The listing builds one solid part. Answer for the finished solid, in the listing's coordinates (mm). A direction names the side the tool comes from. Round coordinates to 2 decimals unless told otherwise and drop trailing zeros. Loops run counter-clockwise (first coordinate to the right, second up) from the corner with the lowest first, then second, coordinate; pieces in that order, holes last. Notation, with made-up numbers: (3, 86.25) - (19, 86.25) arc R19 ccw to (19, 102.25) - close; hole circle Ø1 at (7, -36.75). An arc over 180 degrees is marked (long way). One line per item, written item: value.
```python
from build123d import *

# Parameters (mm, degrees)
SKETCH1_W           = 155
SKETCH1_H           = 155
SKETCH1_R           = 1.5
SKETCH1_W_2         = 85
SKETCH1_H_2         = 85
BOSS_EXTRUDE1_DEPTH = 8
SKETCH3_W           = 128
SKETCH3_H           = 128
CUT_EXTRUDE2_DEPTH  = 2.85
FILLET1_R           = 3
SKETCH4_R           = 2.5
CUT_EXTRUDE3_DEPTH  = 2.5
SKETCH5_R           = 1.75
CUT_EXTRUDE4_DEPTH  = 23
SKETCH6_R           = 3.35
CUT_EXTRUDE5_DEPTH  = 3.5


with BuildPart() as part:
    # Sketch1 → Boss-Extrude1 (new body)
    with BuildSketch(Plane.XY):
        Rectangle(SKETCH1_W, SKETCH1_H)
        with Locations((-50, 50)):
            Circle(SKETCH1_R, mode=Mode.SUBTRACT)
        with Locations((50, 50)):
            Circle(SKETCH1_R, mode=Mode.SUBTRACT)
        with Locations((50, -50)):
            Circle(SKETCH1_R, mode=Mode.SUBTRACT)
        with Locations((-50, -50)):
            Circle(SKETCH1_R, mode=Mode.SUBTRACT)
        Rectangle(SKETCH1_W_2, SKETCH1_H_2, mode=Mode.SUBTRACT)
    extrude(amount=BOSS_EXTRUDE1_DEPTH)

    # Sketch3 → Cut-Extrude2 (cut)
    with BuildSketch(Plane.XY.offset(8)):
        Rectangle(SKETCH3_W, SKETCH3_H)
    extrude(amount=-CUT_EXTRUDE2_DEPTH, mode=Mode.SUBTRACT)

    # Fillet1
    fillet1_edges = [part.edges().sort_by_distance(p)[0] for p in [
        (77.5, -77.5, 4),
        (-77.5, -77.5, 4),
        (-77.5, 77.5, 4),
        (77.5, 77.5, 4),
    ]]
    fillet(fillet1_edges, radius=FILLET1_R)

    # Sketch4 → Cut-Extrude3 (cut)
    with BuildSketch(Plane(origin=(0, 0, 5.15), x_dir=(-1, 0, 0), z_dir=(0, 0, -1))):
        with Locations((-50, 50)):
            Circle(SKETCH4_R)
        with Locations((50, 50)):
            Circle(SKETCH4_R)
        with Locations((50, -50)):
            Circle(SKETCH4_R)
        with Locations((-50, -50)):
            Circle(SKETCH4_R)
    extrude(amount=CUT_EXTRUDE3_DEPTH, mode=Mode.SUBTRACT)

    # Sketch5 → Cut-Extrude4 (cut)
    with BuildSketch(Plane.XY.offset(8)):
        with Locations((0, 69.431322576)):
            Circle(SKETCH5_R)
        with Locations((-69.610191061, 69.610191061)):
            Circle(SKETCH5_R)
        with Locations((69.431322576, 0)):
            Circle(SKETCH5_R)
        with Locations((69.610191061, 69.610191061)):
            Circle(SKETCH5_R)
        with Locations((0, -69.431322576)):
            Circle(SKETCH5_R)
        with Locations((69.610191061, -69.610191061)):
            Circle(SKETCH5_R)
        with Locations((-69.431322576, 0)):
            Circle(SKETCH5_R)
        with Locations((-69.610191061, -69.610191061)):
            Circle(SKETCH5_R)
    extrude(amount=-CUT_EXTRUDE4_DEPTH, mode=Mode.SUBTRACT)

    # Sketch6 → Cut-Extrude5 (cut)
    with BuildSketch(Plane(origin=(0, 0, 0), x_dir=(-1, 0, 0), z_dir=(0, 0, -1))):
        with Locations((-69.610191061, 69.610191061)):
            Circle(SKETCH6_R)
        with Locations((69.610191061, 69.610191061)):
            Circle(SKETCH6_R)
        with Locations((69.610191061, -69.610191061)):
            Circle(SKETCH6_R)
        with Locations((-69.610191061, -69.610191061)):
            Circle(SKETCH6_R)
        with Locations((-69.431322576, 0)):
            Circle(SKETCH6_R)
        with Locations((0, 69.431322576)):
            Circle(SKETCH6_R)
        with Locations((69.431322576, 0)):
            Circle(SKETCH6_R)
        with Locations((0, -69.431322576)):
            Circle(SKETCH6_R)
    extrude(amount=-CUT_EXTRUDE5_DEPTH, mode=Mode.SUBTRACT)


solid = part.part
```
1) For a pull along Y with two mould halves and no side action, classify faces 4 (the flat face through (-1.4, -70.9, 3.5)), 5 (the flat face through (-1, -77.5, 4)), 6 (the flat face through (-77.5, -1, 4)) as released by +Y, released by -Y, zero draft, split by the parting line, or undercut.
Final values:
face 4: undercut
face 5: released by -Y
face 6: zero draft
2) A cutting plane is placed at C-C on x = 55. Give the vertices of the cut face in (y, z).
Final values:
outline: (-77.5, 0) - (77.5, 0) - (77.5, 8) - (64, 8) - (64, 5.15) - (-64, 5.15) - (-64, 8) - (-77.5, 8) - close
3) Consider L1, parallel to Y at x = -50, z = 1.85; L2, parallel to Y at x = 41.5, z = 3. Determine where each line is inside the solid, lowest interval first.
Final values:
L1: -77.5 to -51.5, -48.5 to 48.5, 51.5 to 77.5
L2: -77.5 to -42.5, 42.5 to 77.5
4) A cutting plane is placed at A-A on y = 29. Give the vertices of the cut face in (x, z), and give its area (3 significant figures).
Final values:
outline: (-77.5, 0) - (-42.5, 0) - (-42.5, 5.15) - (-64, 5.15) - (-64, 8) - (-77.5, 8) - close; (42.5, 0) - (77.5, 0) - (77.5, 8) - (64, 8) - (64, 5.15) - (42.5, 5.15) - close
area: 437 mm2
5) For faces 1 (the flat face through (-1, -42.5, 3)), 2 (the cylindrical face through (0.73, 66.16, 1.73)), 3 (the flat face through (50, 48, 2.65)), determine the directions among +Z, -Z, +X, -X, +Y, -Y from which every point of the face is accessible in a straight line to the end or side of a thin tool.
Final values:
face 1: +Z, -Z
face 2: -Z
face 3: +Z
6) Each of these flat-tipped pins is pushed along its axis until it touches: pin 1 Ø8 at (x, y) = (-50, 50) entering from +Z; pin 2 Ø6 at (x, y) = (69.61, -69.61) entering from -Z. Where does it stop, or does it pass through?
Final values:
pin 1: z = 5.15
pin 2: z = 3.5
